```python
from build123d import *

# Parameters (mm, degrees)
F0_R     = 32.5
F1_DEPTH = 30
F2_R     = 31.75
F3_DEPTH = 29
F4_R     = 5
F5_R     = 2.5


with BuildPart() as f1:
    # F0 (on Top) → F1 (new body)
    with BuildSketch(Plane.XY):
        Circle(F0_R)
    extrude(amount=F1_DEPTH)

    # F2 (on face) → F3 (cut)
    with BuildSketch(Plane.XY.offset(30)):
        Circle(F2_R)
    extrude(amount=-F3_DEPTH, mode=Mode.SUBTRACT)

    # F4
    f4_edges = [f1.edges().sort_by_distance(p)[0] for p in [
        (-31.75, 0, 1),
    ]]
    fillet(f4_edges, radius=F4_R)

    # F5
    f5_edges = [f1.edges().sort_by_distance(p)[0] for p in [
        (-32.5, 0, 0),
    ]]
    fillet(f5_edges, radius=F5_R)


solid = f1.part
```
Geometry: final body of the model. Coordinates: model frame, mm. A direction names the side the tool comes from. Give positions to 0.01 mm unless a question says otherwise; leave off trailing zeros. Loops run counter-clockwise (first coordinate to the right, second up) from the corner with the lowest first, then second, coordinate; pieces in that order, holes last. Notation, with made-up numbers: (33.25, -35.5) -> (80.25, -35.5) arc R32 cw to (80.25, -1.5) -> close; hole circle Ø6 at (45, 4.25). An arc over 180 degrees is marked (long way). Use one line per item in the form item = value.
Item 1: Section query C-C on z = 15.25. Output: boundary loops of the cut face in (x, y).
A:
outline = circle Ø65 at (0, 0); hole circle Ø63.5 at (0, 0)
Item 2: Pin query (flat end, axial travel): P1, Ø6, axis at x = 0, z = 16.5, coming from the +Y side; P2, Ø8, axis at x = -14, y = -18.5, coming from the +Z side; P3, Ø10, axis at x = 10.5, z = 19, coming from the -Y side. Return the tip coordinate at first contact, or that it passes through.
A:
P1 = 32.5
P2 = 1.02
P3 = -32.03
Item 3: Access query for faces 1 (the face through (7.1, -31.1, 30)), 2 (the face through (-6.883, -30.995, 18.168)). Directions: +Z, -Z, +X, -X, +Y, -Y. A direction counts if a zero-diameter tool reaches every point of the face in a straight line with its end or side. Return the directions, or none.
A:
face_1 = +Z, +X, -X, +Y, -Y
face_2 = +Z
Item 4: Line query: probe 1 along Y at (x, z) = (0, 11); probe 2 along Z at (x, y) = (9.5, 3.5); probe 3 along Y at (x, z) = (26, 5.75). Output: solid intervals per line, ascending.
A:
probe_1 = -32.5 to -31.75, 31.75 to 32.5
probe_2 = 0 to 1
probe_3 = -19.5 to -18.21, 18.21 to 19.5
Item 5: Draft query along X for faces 3 (the face through (0, 0, 1)), 4 (the face through (31, 9.76, 16.06)), 5 (the face through (0, 0, 0)). Return one class per face: pulls with the +X half, pulls with the -X half, needs draft (parallel to the pull), parting line crosses it, or undercut.
A:
face_3 = undercut
face_4 = parting line crosses it
face_5 = needs draft
Item 6: Section query A-A on y = 0. Output: boundary loops of the cut face in (x, z), and give its area (3 significant figures).
A:
outline = (-32.5, 2.5) arc R2.5 ccw to (-30, 0) -> (30, 0) arc R2.5 ccw to (32.5, 2.5) -> (32.5, 30) -> (31.75, 30) -> (31.75, 6) arc R5 cw to (26.75, 1) -> (-26.75, 1) arc R5 cw to (-31.75, 6) -> (-31.75, 30) -> (-32.5, 30) -> close
area = 117 mm^2
